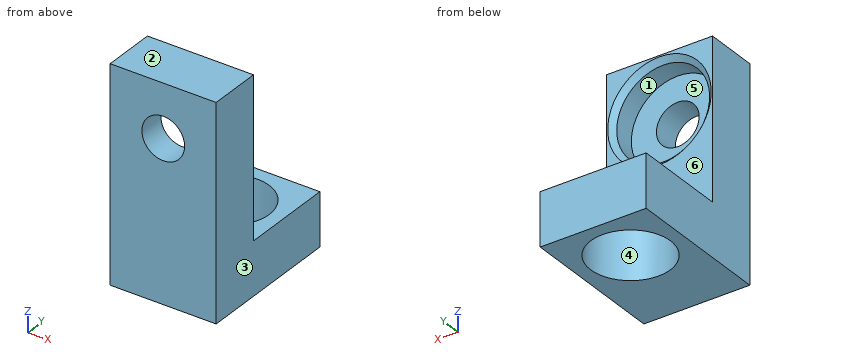
from build123d import *

# Parameters (mm, degrees)
SKETCH1_R           = 4.7625
BOSS_EXTRUDE1_DEPTH = 6.35
SKETCH2_W           = 12.676867833
SKETCH2_H           = 6.35
BOSS_EXTRUDE2_DEPTH = 19.05


with BuildPart() as part:
    # Sketch1 → Boss-Extrude1 (new body)
    with BuildSketch(Plane.XY):
        Polygon((-6.326867833, 0), (-6.326867833, -11.303), (6.35, -11.303), (6.35, 0), (6.35, 6.35), (-6.326867833, 6.35), align=None)
        Circle(SKETCH1_R, mode=Mode.SUBTRACT)
    extrude(amount=BOSS_EXTRUDE1_DEPTH)

    # Sketch2 → Boss-Extrude2 (add)
    with BuildSketch(Plane.XY.offset(6.35)):
        with Locations((0.011566083, -8.128)):
            Rectangle(SKETCH2_W, SKETCH2_H)
    extrude(amount=BOSS_EXTRUDE2_DEPTH)

    # Sketch7 → CBORE for #10 Binding Head Machine Screw1 (revolve, cut)
    with BuildSketch(Plane(origin=(0.023132167, -4.953, 19.05), x_dir=(0, 0, 1), z_dir=(1, 0, 0))):
        Polygon((0, 0), (0, 6.35), (2.5527, 6.35), (2.5527, 3.1242), (5.55625, 3.1242), (5.55625, 0.635), (6.19125, 0), align=None)
    revolve(axis=Axis((0.023132167, 1.397, 19.05), (0, -1, 0)), mode=Mode.SUBTRACT)


solid = part.part
For this review, take the finished solid that the model builds, in its own axes (mm). Face numbers are marked on the shaded views. A direction names the side the tool comes from. Coordinates: 2 decimals unless noted, no trailing zeros. Loops run counter-clockwise (first coordinate to the right, second up) from the corner with the lowest first, then second, coordinate; pieces in that order, holes last. Notation, with made-up numbers: (37.5, 54) - (73.5, 54) arc R7 cw to (73.5, 58) - close; hole circle Ø5 at (-36, 17). An arc over 180 degrees is marked (long way). Use a Markdown table: item, result. Add a question column.
Item 1: For line 1 (X direction, y = -7.25, z = 19.05); line 2 (X direction, y = -10.25, z = 19.05); line 3 (Y direction, x = 0, z = 1.75), list the stretches that pass through material, from the lowest coordinate up.
Item 2: Mouldability with a two-part tool opening along X and no side actions: class the marked faces 1, 2 and 3 as pulls with the +X half, pulls with the -X half, needs draft (parallel to the pull), parting line crosses it, or undercut.
Item 3: Insertion check: pin 1 Ø3.5 at (x, y) = (0.5, 2.5) entering from +Z. The pin has a flat end and moves straight along its axis. Give the tip position at first contact, or say it passes through.
Item 4: We need section B-B (y = 0). Give the boundary of the cut face in (x, z).
Item 5: We need section A-A (z = 19.05). Give the boundary of the cut face in (x, y).
Item 6: We need section D-D (x = -1.5). Give the number of separate pieces and of enclosed holes in the cut face, and give its area (3 significant figures).
Item 7: Tool access review of the marked faces 4, 5 and 6: name each direction out of +Z, -Z, +X, -X, +Y, -Y from which nothing blocks a thin tool from reaching the whole face with its end or side.
Results list:
| question | item | result |
|---|---|---|
| 1 | line 1 | x = -6.33 to -5.53, 5.58 to 6.35 |
| 1 | line 2 | x = -6.33 to -2.53, 2.58 to 6.35 |
| 1 | line 3 | y = -11.3 to -4.76, 4.76 to 6.35 |
| 2 | face 1 | undercut |
| 2 | face 2 | needs draft |
| 2 | face 3 | pulls with the +X half |
| 3 | pin 1 | passes through |
| 4 | outline | (-6.33, 0) - (-4.76, 0) - (-4.76, 6.35) - (-6.33, 6.35) - close; (4.76, 0) - (6.35, 0) - (6.35, 6.35) - (4.76, 6.35) - close |
| 5 | outline | (-6.33, -11.3) - (-2.53, -11.3) - (-2.53, -8.08) - (-5.53, -8.08) - (-5.53, -5.59) - (-6.17, -4.95) - (-6.33, -4.95) - close; (2.58, -11.3) - (6.35, -11.3) - (6.35, -4.95) - (6.21, -4.95) - (5.58, -5.59) - (5.58, -8.08) - (2.58, -8.08) - close |
| 6 | separate pieces | 3 |
| 6 | enclosed holes | 0 |
| 6 | area | 129 mm^2 |
| 7 | face 4 | +Z, -Z |
| 7 | face 5 | +Y |
| 7 | face 6 | +Z, +X, -X, +Y |
